Here's how the part is built. I have some questions about the finished solid (model axes, mm). Face numbers are marked on the shaded views. Give positions to 0.01 mm unless a question says otherwise; leave off trailing zeros. Write each loop counter-clockwise with the first axis right and the second up, starting at its lowest first coordinate (ties: lowest second). Pieces come first, ordered by that corner, then holes. Notation, with made-up numbers: (-25, -5) -> (-12, -5) arc R18 ccw to (-12, 4) -> close; hole circle Ø5 at (-34, 47.25). An arc over 180 degrees is marked (long way). Answer as CSV lines item,"result". Start each with the question number.
from build123d import *

# Parameters (mm, degrees)
SKETCH1_W           = 5.5
SKETCH1_H           = 7
BOSS_EXTRUDE1_DEPTH = 5
BOSS_EXTRUDE2_DEPTH = 5.5
SKETCH4_R           = 2.55
CUT_EXTRUDE1_DEPTH  = 11.210288928
SKETCH5_R           = 2.499369643
CUT_EXTRUDE2_DEPTH  = 4


with BuildPart() as part:
    # Sketch1 → Boss-Extrude1 (new body)
    with BuildSketch(Plane.XY):
        with Locations((2.75, 3.5)):
            Rectangle(SKETCH1_W, SKETCH1_H)
    extrude(amount=BOSS_EXTRUDE1_DEPTH)

    # Sketch3 → Boss-Extrude2 (add)
    with BuildSketch(Plane(origin=(5.5, 0, 0), x_dir=(0, 0, -1), z_dir=(1, 0, 0))):
        with BuildLine():
            Line((0, 7), (0, 0))
            ThreePointArc((0, 0), (3.5, 3.5), (0, 7))
        make_face()
    extrude(amount=-BOSS_EXTRUDE2_DEPTH)

    # Sketch4 → Cut-Extrude1 (cut, through all)
    with BuildSketch(Plane.ZY):
        with Locations((-0.797128345, 3.5)):
            Circle(SKETCH4_R)
    extrude(amount=-CUT_EXTRUDE1_DEPTH, mode=Mode.SUBTRACT)

    # Sketch5 → Cut-Extrude2 (cut)
    with BuildSketch(Plane.XY.offset(5)):
        with Locations((2.75, 3.5)):
            Circle(SKETCH5_R)
    extrude(amount=-CUT_EXTRUDE2_DEPTH, mode=Mode.SUBTRACT)


solid = part.part
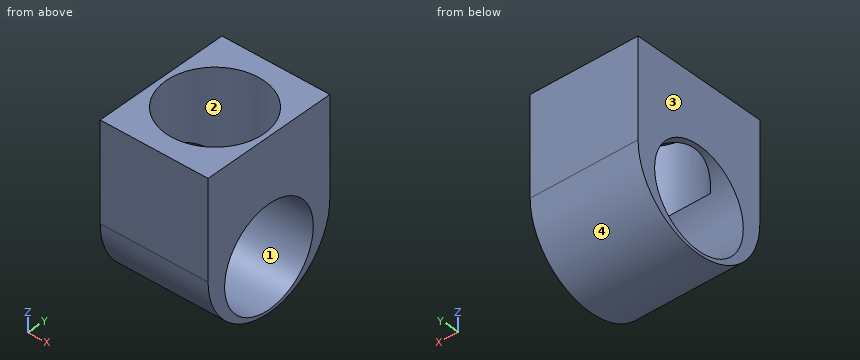
Item 1: If we section it at C-C (x = 2.75): Please give me the cut outline in (y, z).
Item 2: We'd pull the mould along Y, two halves only. Please class the marked faces 1, 2, 3 and 4: released by +Y, released by -Y, zero draft, split by the parting line, or undercut.
Item 3: If we section it at B-B (z = 1.5): Please give me the cut outline in (x, y).
Item 4: If we section it at A-A (y = 3.5): Please give me the cut outline in (x, z), and give its area (3 significant figures).
Item 5: If we section it at D-D (y = 2): Please give me the cut outline in (x, z).
Item 6: If I drill on line 1 (X direction, y = 3.5, z = 3.25); line 2 (Y direction, x = 3.3, z = 0.75); line 3 (X direction, y = 4.25, z = 4.25), over which ranges is the centre line in solid material (lowest first)? Write a range as [from, to].
Item 7: I'm going to push flat-ended pins straight in: pin 1 (0.8 mm diameter, centred on x = 3, y = 1.5, fed in from +Z); pin 2 (4 mm diameter, centred on y = 5.5, z = 0, fed in from +X). Where does each tip first touch, or does it pass through?
Final values:
1,outline,"(0, 0) arc R3.5 ccw to (7, 0) -> (7, 5) -> (6, 5) -> (6, 1) -> (5.31, 1) arc R2.55 cw (long way) to (1.69, 1) -> (1, 1) -> (1, 5) -> (0, 5) -> close"
2,face 1,"undercut"
2,face 2,"undercut"
2,face 3,"zero draft"
2,face 4,"split by the parting line"
3,outline,"(0, 0) -> (5.5, 0) -> (5.5, 2.39) -> (4.99, 2.39) arc R2.5 cw to (0.51, 2.39) -> (0, 2.39) -> close; (0, 4.61) -> (0.51, 4.61) arc R2.5 cw to (4.99, 4.61) -> (5.5, 4.61) -> (5.5, 7) -> (0, 7) -> close"
4,outline,"(0, -3.5) -> (5.5, -3.5) -> (5.5, -3.35) -> (0, -3.35) -> close; (0, 1.75) -> (0.25, 1.75) -> (0.25, 5) -> (0, 5) -> close; (5.25, 1.75) -> (5.5, 1.75) -> (5.5, 5) -> (5.25, 5) -> close"
4,area,"2.47 mm2"
5,outline,"(0, -3.16) -> (5.5, -3.16) -> (5.5, -2.86) -> (0, -2.86) -> close; (0, 1.27) -> (0.75, 1.27) -> (0.75, 5) -> (0, 5) -> close; (4.75, 1.27) -> (5.5, 1.27) -> (5.5, 5) -> (4.75, 5) -> close"
6,line 1,"[0, 0.25], [5.25, 5.5]"
6,line 2,"[0, 1.47], [5.53, 7]"
6,line 3,"[0, 0.37], [5.13, 5.5]"
7,pin 1,"z = 1"
7,pin 2,"x = 5.5"
